Here's the drawing with two shaded views (mm, measured from the low corner). I have some questions. Coordinates: 2 decimals unless noted, no trailing zeros. Loops run counter-clockwise (first coordinate to the right, second up) from the corner with the lowest first, then second, coordinate; pieces in that order, holes last. Notation, with made-up numbers: (1, 38.25) - (14, 38.25) arc R6 ccw to (14, 49.25) - close; hole circle Ø8 at (45, -26.5). An arc over 180 degrees is marked (long way). One line per item, written item: value. Start each with the question number.
(1) I'm going to push flat-ended pins straight in: P1, Ø8, axis at x = 5, y = 27, coming from the +Z side; P2, Ø8, axis at y = 15, z = 9, coming from the -X side; P3, Ø2, axis at x = 15.5, y = 9.5, coming from the +Z side. Where does each tip first touch, or does it pass through?
(2) If we section it at A-A on y = 17: Write out the boundary of the cut face in (x, z), then the cut area to 3 significant figures.
(3) If we section it at B-B on y = 9.5: Write out the boundary of the cut face in (x, z).
(4) If we mould it in two halves opening along X, with no side actions, what happens to the marked faces 1, 2 and 3? For each: pulls with the +X half, pulls with the -X half, needs draft (parallel to the pull), parting line crosses it, or undercut.
(5) If I drill on line 1 along Y through (x, z) = (16, 6.5); line 2 along Z through (x, y) = (12.7, 7.5), over which ranges is the centre line in solid material (lowest first)? Write a range as from..to.
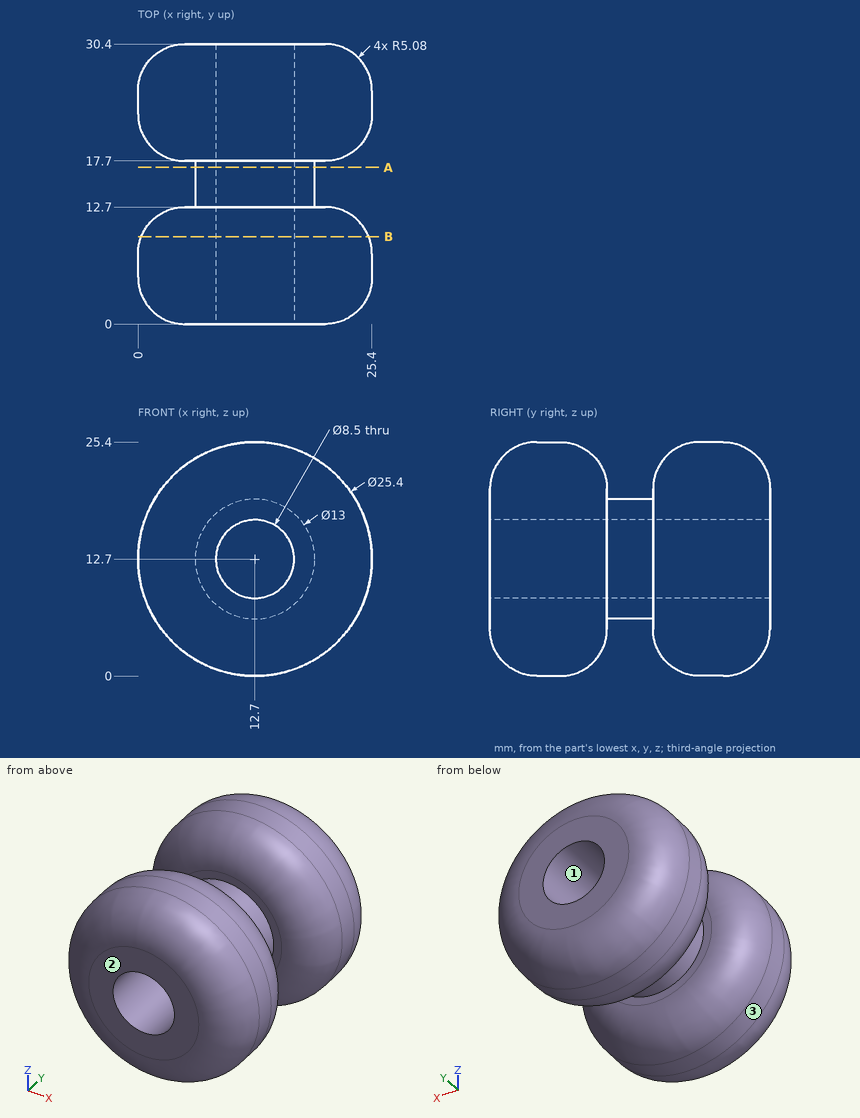
Values:
1. P1: stops at z = 24.77
1. P2: stops at x = 1.73
1. P3: stops at z = 25.09
2. outline: circle Ø13 at (12.7, 12.7); hole circle Ø8.5 at (12.7, 12.7)
2. area: 76.0 mm2
3. outline: circle Ø24.68 at (12.7, 12.7); hole circle Ø8.5 at (12.7, 12.7)
4. face 1: undercut
4. face 2: needs draft
4. face 3: parting line crosses it
5. line 1: y = 0..12.7, 17.7..30.4
5. line 2: z = 0..8.45, 16.95..25.4
